```python
from build123d import *

# Parameters (mm, degrees)
CHAMFER1_SIZE      = 0.5
CUT_EXTRUDE1_DEPTH = 2.4


with BuildPart() as part:
    # Sketch1 → Revolve1 (revolve)
    with BuildSketch(Plane.XY):
        with BuildLine():
            Line((0, 0), (0, 3.5))
            ThreePointArc((0, 3.5), (-0.146446609, 3.853553391), (-0.5, 4))
            Line((-0.5, 4), (-4, 4))
            Line((-4, 4), (-4, 2.5))
            Line((-4, 2.5), (-19, 2.5))
            Line((-19, 2.5), (-19, 2))
            Line((-19, 2), (-27, 2))
            Line((-27, 2), (-27, 0))
            Line((-27, 0), (0, 0))
        make_face()
    revolve(axis=Axis((0, 0, 0), (1, 0, 0)))

    # Chamfer1
    chamfer1_edges = [part.edges().sort_by_distance(p)[0] for p in [
        (-27, -2, 0),
    ]]
    chamfer(chamfer1_edges, length=CHAMFER1_SIZE)

    # Sketch2 → Cut-Extrude1 (cut)
    with BuildSketch(Plane(origin=(0, 0, 0), x_dir=(0, 0, -1), z_dir=(1, 0, 0))):
        Polygon((1.732050808, 0), (0.866025404, 1.5), (-0.866025404, 1.5), (-1.732050808, 0), (-0.866025404, -1.5), (0.866025404, -1.5), align=None)
    extrude(amount=-CUT_EXTRUDE1_DEPTH, mode=Mode.SUBTRACT)


solid = part.part
```
Geometry check sheet. Reference: the model listing, model coordinates, mm. A direction names the side the tool comes from. Round coordinates to 2 decimals unless told otherwise and drop trailing zeros. Order: outer loops, then holes, each group sorted by start corner. A loop starts at its lowest first (then second) coordinate and runs counter-clockwise, first axis right, second up. Notation, with made-up numbers: (53, 66) - (88, 66) arc R21 ccw to (88, 75) - close; hole circle Ø1 at (-1.5, -17). An arc over 180 degrees is marked (long way). Use a Markdown table: item, result. Add a question column.
(1) Sectioned sample at A-A, the plane z = 0. Enter the section's corners in (x, y).
(2) Material ranges on line 1 along X through (y, z) = (2, -2); line 2 along Y through (x, z) = (-1.25, 0.5); line 3 along Y through (x, z) = (-14.5, -1.5), recorded low to high. Write a range as [from, to].
(3) Sectioned sample at B-B, the plane x = -10. Enter the section's corners in (y, z), and give its area (3 significant figures).
(4) Depth check by flat-ended pin: pin 1 (1.5 mm diameter, centred on x = -24, y = 1.5, fed in from -Z); pin 2 (4 mm diameter, centred on x = -4.5, z = 3, fed in from +Y); pin 3 (3 mm diameter, centred on x = -19, y = -2.5, fed in from -Z). Enter the tip coordinate at first touch or a pass-through.
(5) Tool access check on faces 1 (the flat face through (-1, -1.5, 0)), 2 (the cylindrical face through (-2.274, -0.867, -3.905)), 3 (the cylindrical face through (-11.6, -0.54, -2.44)). Record the directions out of +Z, -Z, +X, -X, +Y, -Y that give a thin tool (end or side, any length) a straight path to the whole face; none if there is none.
(6) Release check for a two-part mould opening along Z. For faces 4 (the flat face through (-1.183, -0.74, 1.305)), 5 (the flat face through (-4, 2, 2)), 6 (the cylindrical face through (-23, 0, -2)), 7 (the flat face through (-1.183, -0.76, -1.293)) record: pulls with the +Z half, pulls with the -Z half, needs draft (parallel to the pull), parting line crosses it, or undercut.
Answers below:
| question | item | result |
|---|---|---|
| 1 | outline | (-27, -1.5) - (-26.5, -2) - (-19, -2) - (-19, -2.5) - (-4, -2.5) - (-4, -4) - (-0.5, -4) arc R0.5 ccw to (0, -3.5) - (0, -1.5) - (-2.4, -1.5) - (-2.4, 1.5) - (0, 1.5) - (0, 3.5) arc R0.5 ccw to (-0.5, 4) - (-4, 4) - (-4, 2.5) - (-19, 2.5) - (-19, 2) - (-26.5, 2) - (-27, 1.5) - close |
| 2 | line 1 | [-4, 0] |
| 2 | line 2 | [-3.97, -1.5], [1.5, 3.97] |
| 2 | line 3 | [-2, 2] |
| 3 | outline | circle Ø5 at (0, 0) |
| 3 | area | 19.6 mm² |
| 4 | pin 1 | z = -1.85 |
| 4 | pin 2 | y = 3.86 |
| 4 | pin 3 | z = -2.29 |
| 5 | face 1 | +X |
| 5 | face 2 | +X, -X |
| 5 | face 3 | -X |
| 6 | face 4 | undercut |
| 6 | face 5 | needs draft |
| 6 | face 6 | parting line crosses it |
| 6 | face 7 | undercut |
